Source: CAD feature listing. Evaluate the final solid. Frame: model axes, mm. Round coordinates to 2 decimals unless told otherwise and drop trailing zeros. Loops run counter-clockwise (first coordinate to the right, second up) from the corner with the lowest first, then second, coordinate; pieces in that order, holes last.
(1) Material intervals for probe 1 along Z at (x, y) = (-31.3, 4.5); probe 2 along Z at (x, y) = (-10, 1.75); probe 3 along Z at (x, y) = (-8.5, 4.5), sorted ascending.
(2) First-contact query: pin 1 Ø2.5 at (y, z) = (4.5, -10.35) entering from -X; pin 2 Ø1.7 at (x, z) = (-25.5, -43) entering from -Y. Flat tips, straight axial feed; report the tip coordinate or a pass-through.
(3) Section A-A, the plane z = -136.5. Return the cut outline in (x, y), plus the area to 3 significant figures.
(4) Section B-B, the plane z = -10.35. Count the separate pieces of the cut face and the enclosed holes in it, plus the area to 3 significant figures.
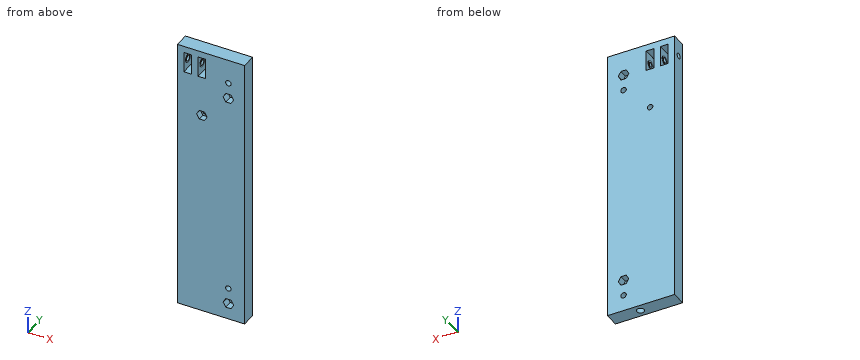
Autodesk Inventor part; units mm, degrees
ref_plane "YZ Plane" through (0, 0, 0) normal (1, 0, 0) x (0, 1, 0)
ref_plane "XZ Plane" through (0, 0, 0) normal (0, 1, 0) x (-1, 0, 0)
ref_plane "XY Plane" through (0, 0, 0) normal (0, 0, 1) x (1, 0, 0)
sketch "Sketch1" plane through (0, 0, 0) normal (0, 1, 0) x (-1, 0, 0)
  line L0 (0, 0) -> (41.5, 0)
  line L1 (41.5, 0) -> (41.5, -170)
  line L2 (41.5, -170) -> (0, -170)
  line L3 (0, -170) -> (0, 0)
  dimension "d0" = 41.5
  dimension "d1" = 170
extrude "Extrusion1" add sketch "Sketch1" along normal blind 9
sketch "Sketch2" plane through (0, 9, 0) normal (0, 1, 0) x (1, 0, 0)
  circle A0 centre (-10, 15) radius 3.25 construction
  line L0 (-41.5, 0) -> (0, 0)
  line L1 (0, 0) -> (0, 170)
  line L2 (-13.25, 15) -> (-11.625, 17.8146)
  line L3 (-11.625, 17.8146) -> (-8.375, 17.8146)
  line L4 (-8.375, 17.8146) -> (-6.75, 15)
  line L5 (-6.75, 15) -> (-8.375, 12.1854)
  line L6 (-8.375, 12.1854) -> (-11.625, 12.1854)
  line L7 (-11.625, 12.1854) -> (-13.25, 15)
  circle A1 centre (-10, 150) radius 3.25 construction
  line L8 (-13.25, 150) -> (-11.625, 152.8146)
  line L9 (-11.625, 152.8146) -> (-8.375, 152.8146)
  line L10 (-8.375, 152.8146) -> (-6.75, 150)
  line L11 (-6.75, 150) -> (-8.375, 147.1854)
  line L12 (-8.375, 147.1854) -> (-11.625, 147.1854)
  line L13 (-11.625, 147.1854) -> (-13.25, 150)
  line L14 (0, 170) -> (-41.5, 170)
  circle A2 centre (-10, 15) radius 1.7 construction
  circle A3 centre (-10, 150) radius 1.7 construction
  dimension "d7" = 6.5
  dimension "d10" = 6.5
  dimension "d23" = 135
  dimension "d24" = 15
  dimension "d25" = 10
  dimension "d28" = 3.4
  dimension "d29" = 3.4
extrude "Extrusion2" cut sketch "Sketch2" against normal blind 5
sketch "Sketch3" plane through (0, 0, 0) normal (0, -1, 0) x (1, 0, 0)
  circle A0 centre (-10, -25) radius 3.25 construction
  line L0 (0, 0) -> (-41.5, 0)
  line L1 (-41.5, 0) -> (-41.5, -170)
  line L2 (-11.6286, -27.8125) -> (-13.25, -24.9958)
  line L3 (-13.25, -24.9958) -> (-11.6214, -22.1833)
  line L4 (-11.6214, -22.1833) -> (-8.3714, -22.1875)
  line L5 (-8.3714, -22.1875) -> (-6.75, -25.0042)
  line L6 (-6.75, -25.0042) -> (-8.3786, -27.8167)
  line L7 (-8.3786, -27.8167) -> (-11.6286, -27.8125)
  circle A1 centre (-10, -160) radius 3.25 construction
  line L8 (-6.75, -160) -> (-8.375, -162.8146)
  line L9 (-8.375, -162.8146) -> (-11.625, -162.8146)
  line L10 (-11.625, -162.8146) -> (-13.25, -160)
  line L11 (-13.25, -160) -> (-11.625, -157.1854)
  line L12 (-11.625, -157.1854) -> (-8.375, -157.1854)
  line L13 (-8.375, -157.1854) -> (-6.75, -160)
  line L14 (0, -170) -> (0, 0)
  dimension "d15" = 6.5
  dimension "d18" = 6.5
  dimension "d16" = 25
  dimension "d19" = 135
  dimension "d26" = 10
  dimension "d27" = 10
extrude "Extrusion3" cut sketch "Sketch3" against normal blind 5
sketch "Sketch5" plane through (0, 9, 0) normal (0, 1, 0) x (1, 0, 0)
  circle A0 centre (-10, 15) radius 1.7
  line L0 (0, 0) -> (0, 170)
  line L1 (-41.5, 0) -> (0, 0)
  circle A1 centre (-10, 150) radius 1.7
  circle A2 centre (-10, 25) radius 1.7
  circle A3 centre (-10, 160) radius 1.7
  dimension "d30" = 3.4
  dimension "d31" = 10
  dimension "d32" = 15
  dimension "d33" = 3.4
  dimension "d34" = 10
  dimension "d35" = 135
  dimension "d36" = 3.4
  dimension "d37" = 25
  dimension "d38" = 3.4
  dimension "d39" = 10
  dimension "d40" = 135
extrude "Extrusion4" cut sketch "Sketch5" against normal through all
sketch "Sketch6" plane through (0, 9, 0) normal (0, 1, 0) x (1, 0, 0)
  line L0 (-37.5, 4) -> (-32.7502, 4)
  line L1 (-32.7502, 4) -> (-32.7502, 16.7)
  line L2 (-32.7502, 16.7) -> (-37.5, 16.7)
  line L3 (-37.5, 16.7) -> (-37.5, 4)
  line L4 (-41.5, 0) -> (0, 0)
  line L5 (-41.5, 170) -> (-41.5, 0)
  line L6 (-28.7502, 4) -> (-24.0002, 4)
  line L7 (-24.0002, 4) -> (-24.0002, 16.7)
  line L8 (-24.0002, 16.7) -> (-28.7502, 16.7)
  line L9 (-28.7502, 16.7) -> (-28.7502, 4)
  line L10 (0, 0) -> (0, 170) construction
  line L11 (-41.5, 170) -> (0, 170)
  line L12 (0, 0) -> (-20, 0) construction
  line L13 (-20, 0) -> (-20, 170) construction
  line L14 (-20, 170) -> (0, 170) construction
  line L15 (0, 170) -> (0, 0)
  circle A0 centre (-26.3752, 41.7) radius 1.7
  dimension "d43" = 4.7498
  dimension "d44" = 12.7
  dimension "d45" = 4
  dimension "d46" = 4
  dimension "d47" = 4.75
  dimension "d48" = 4
  dimension "d49" = 20
  dimension "d50" = 3.4
  dimension "d51" = 25
extrude "Extrusion5" cut sketch "Sketch6" against normal through all contours L3 L2 L1 L0 | L9 L8 L7 L6 | A0
sketch "Sketch7" plane through (0, 0, 0) normal (0, -1, 0) x (1, 0, 0)
  circle A0 centre (-26.3752, -41.7) radius 1.7
  circle A1 centre (-26.3752, -41.7) radius 3.25 construction
  line L0 (-23.1252, -41.7) -> (-24.7502, -44.5146)
  line L1 (-24.7502, -44.5146) -> (-28.0002, -44.5146)
  line L2 (-28.0002, -44.5146) -> (-29.6252, -41.7)
  line L3 (-29.6252, -41.7) -> (-28.0002, -38.8854)
  line L4 (-28.0002, -38.8854) -> (-24.7502, -38.8854)
  line L5 (-24.7502, -38.8854) -> (-23.1252, -41.7)
  point P0 (0, 0)
  dimension "d54" = 6.5
extrude "Extrusion6" cut sketch "Sketch7" against normal blind 4
sketch "Sketch8" plane through (-41.5, 0, -170) normal (-1, 0, 0) x (0, 0, 1)
  circle A0 centre (159.65, 4.5) radius 1.4605
  line L0 (0, 9) -> (170, 9)
  line L1 (170, 0) -> (170, 9)
  dimension "d57" = 2.921
  dimension "d58" = 4.5
  dimension "d59" = 10.35
hole "Hole1" at (-41.5, 4.5, -10.35) direction (1, 0, 0) diameter 2.921 depth 21 counterbore diameter 3.4 counterbore depth 17
sketch "Sketch9" plane through (-24.0002, 9, -16.7) normal (-1, 0, 0) x (0, 0, 1)
  circle A0 centre (6.35, -4.5) radius 1.4605
  circle A1 centre (6.35, -4.5) radius 2.54
  point P0 (16.7, -9)
  dimension "d67" = 5.08
extrude "Extrusion7" add sketch "Sketch9" along normal blind 0.2032
sketch "Sketch10" plane through (-32.7502, 9, -16.7) normal (-1, 0, 0) x (0, 0, 1)
  circle A0 centre (6.35, -4.5) radius 1.7
  circle A1 centre (6.35, -4.5) radius 2.54
  point P0 (16.7, -9)
  dimension "d70" = 5.08
extrude "Extrusion8" add sketch "Sketch10" along normal blind 0.2032
sketch "Sketch11" plane through (-28.7502, 9, -4) normal (1, 0, 0) x (0, 0, -1)
  circle A0 centre (6.35, -4.5) radius 1.7
  circle A1 centre (6.35, -4.5) radius 2.54
  point P0 (-4, -9)
  dimension "d73" = 5.08
extrude "Extrusion9" add sketch "Sketch11" along normal blind 0.2032
sketch "Sketch12" plane through (-37.5, 9, -4) normal (1, 0, 0) x (0, 0, -1)
  circle A0 centre (6.35, -4.5) radius 1.7
  circle A1 centre (6.35, -4.5) radius 2.54
  point P0 (-4, -9)
  dimension "d76" = 5.08
extrude "Extrusion10" add sketch "Sketch12" along normal blind 0.2032
sketch "Sketch14" plane through (0, 0, -170) normal (0, 0, -1) x (-1, 0, 0)
  circle A0 centre (18, 4.5) radius 2.25
  line L0 (41.5, 0) -> (0, 0)
  line L1 (0, 0) -> (0, 9)
  dimension "d82" = 4.5
  dimension "d83" = 4.5
  dimension "d84" = 18
extrude "Extrusion11" cut sketch "Sketch14" against normal blind 40
properties part number "Top cuppler"
Output values:
1. probe 1: z = -170 to -12.05, -8.65 to 0
1. probe 2: z = -170 to -162.81, -157.19 to -151.7, -148.3 to -27.81, -22.19 to -16.7, -13.3 to 0
1. probe 3: z = -170 to -162.81, -157.19 to -152.81, -147.19 to -27.82, -22.19 to -17.81, -12.19 to 0
2. pin 1: stops at x = -20.5
2. pin 2: stops at y = 4
3. outline: (-41.5, 0) - (0, 0) - (0, 9) - (-41.5, 9) - close; hole circle Ø4.5 at (-18, 4.5)
3. area: 358 mm2
4. separate pieces: 5
4. enclosed holes: 0
4. area: 252 mm2
